from build123d import *

# Parameters (mm, degrees)
SKETCH_1_W          = 7.7
SKETCH_1_H          = 5.6
EXTRUDE_1_DEPTH     = 3
SKETCH_2_R          = 0.5
CUT_EXTRUDE_2_DEPTH = 8.8
SKETCH_3_W          = 6.7
SKETCH_3_H          = 2
CUT_EXTRUDE_3_DEPTH = 5
EXTRUDE_2_DEPTH     = 5


with BuildPart() as part:
    # Эскиз1 → Бобышка-Вытянуть1 (new body)
    with BuildSketch(Plane.XY):
        Rectangle(SKETCH_1_W, SKETCH_1_H)
    extrude(amount=EXTRUDE_1_DEPTH)

    # Эскиз2 → Вырез-Вытянуть2 (cut)
    with BuildSketch(Plane.XY.offset(3)):
        with Locations((0, -2.8)):
            Circle(SKETCH_2_R)
    extrude(amount=-CUT_EXTRUDE_2_DEPTH, mode=Mode.SUBTRACT)

    # Эскиз3 → Вырез-Вытянуть3 (cut)
    with BuildSketch(Plane.XZ.offset(2.8)):
        with Locations((0, 1.5)):
            Rectangle(SKETCH_3_W, SKETCH_3_H)
    extrude(amount=-CUT_EXTRUDE_3_DEPTH, mode=Mode.SUBTRACT)

    # Эскиз4 → Бобышка-Вытянуть2 (add)
    with BuildSketch(Plane.XZ.offset(-2.2)):
        Polygon((-3.35, 2.5), (-2.35, 0.5), (-3.35, 0.5), align=None)
        Polygon((3.35, 2.5), (3.35, 0.5), (2.35, 0.5), align=None)
    extrude(amount=EXTRUDE_2_DEPTH)


solid = part.part
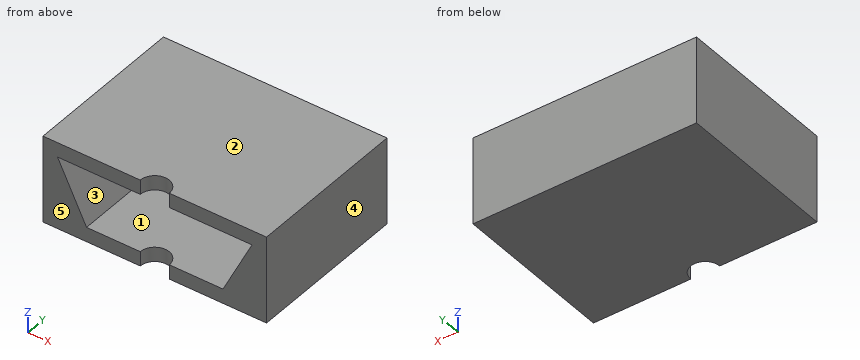
Geometry: final body of the model. Coordinates: model frame, mm. Face numbers are marked on the shaded views. A direction names the side the tool comes from. Give positions to 0.01 mm unless a question says otherwise; leave off trailing zeros. Write each loop counter-clockwise with the first axis right and the second up, starting at its lowest first coordinate (ties: lowest second). Pieces come first, ordered by that corner, then holes.
(1) Access query for the marked faces 1 and 2. Directions: +Z, -Z, +X, -X, +Y, -Y. A direction counts if a zero-diameter tool reaches every point of the face in a straight line with its end or side. Return the directions, or none.
(2) Cut plane C-C, the plane x = 1.5. Return loops of the section in (y, z).
(3) Mould query, pull axis X, two halves, no side actions, for the marked faces 3, 4 and 5. Classes: released by +X, released by -X, zero draft, split by the parting line, or undercut.
(4) Ray query, line 1 (Z direction, x = 2.25, y = -0.9); line 2 (Y direction, x = 0, z = 0.6); line 3 (X direction, y = 0.2, z = 0.8). Return the intervals inside material, ascending.
(5) Cut plane A-A, the plane y = -2. Return loops of the section in (x, z), then the cut area to 3 significant figures.
(6) First-contact query: P1, Ø0.6, axis at x = -1.5, z = 1, coming from the -Y side; P2, Ø2.5, axis at x = 1, y = -1.5, coming from the -Z side. Flat tips, straight axial feed; report the tip coordinate or a pass-through.
(7) Cut plane B-B, the plane z = 1.5. Return loops of the section in (x, y), then the cut area to 3 significant figures.
Values follow:
1. face 1: -Y
1. face 2: +Z, +X, -X, +Y, -Y
2. outline: (-2.8, 0) - (2.8, 0) - (2.8, 3) - (-2.8, 3) - (-2.8, 2.5) - (2.2, 2.5) - (2.2, 0.5) - (-2.8, 0.5) - close
3. face 3: undercut
3. face 4: released by +X
3. face 5: zero draft
4. line 1: z = 0 to 0.5, 2.5 to 3
4. line 2: y = 2.2 to 2.8
4. line 3: x = -3.85 to -2.5, 2.5 to 3.85
5. outline: (-3.85, 0) - (3.85, 0) - (3.85, 3) - (-3.85, 3) - close; hole (-3.35, 2.5) - (-2.35, 0.5) - (2.35, 0.5) - (3.35, 2.5) - close
5. area: 11.7 mm2
6. P1: stops at y = 2.2
6. P2: stops at z = 0
7. outline: (-3.85, -2.8) - (-2.85, -2.8) - (-2.85, 2.2) - (2.85, 2.2) - (2.85, -2.8) - (3.85, -2.8) - (3.85, 2.8) - (-3.85, 2.8) - close
7. area: 14.6 mm2
